Print and shaded views of the part. All mm, measured from the part's lowest x, y and z. A direction names the side the tool comes from. Round coordinates to 2 decimals unless told otherwise and drop trailing zeros. Write each loop counter-clockwise with the first axis right and the second up, starting at its lowest first coordinate (ties: lowest second). Pieces come first, ordered by that corner, then holes. Notation, with made-up numbers: (5, -5) - (22, -5) arc R15 ccw to (22, 18) - close; hole circle Ø10 at (56, 84). An arc over 180 degrees is marked (long way). Put each result on its own line as item: value. Start each with the question number.
Item 1: Drill centre lines: line 1 (X direction, y = 5.25, z = 1.25); line 2 (Z direction, x = 8, y = 4.25) (3 decimals); line 3 (Y direction, x = 5.25, z = 7.25). Where is each one in solid material? Low to high. Write a range as from..to.
Item 2: 3-axis set-ups, long thin cutter, end or side, ignore diameter. For the marked faces 1 and 2: which of +Z, -Z, +X, -X, +Y, -Y reach the whole face in a straight line?
Item 3: Cut at C-C (z = 2.75). Give the cut face in (x, y).
Item 4: Cut at D-D (z = 13). Give the cut face in (x, y) (3 decimals), and give its area (3 significant figures).
Item 5: Cut at A-A (x = 5.08). Give the cut face in (y, z) (3 decimals), and give its area (3 significant figures).
Item 6: Pin check, flat tips, straight feed: pin 1 Ø1.5 at (y, z) = (6, 7.5) entering from -X; pin 2 Ø6 at (x, y) = (3, 8.5) entering from +Z (3 decimals); pin 3 Ø1.5 at (y, z) = (7, 3) entering from +X; pin 4 Ø6 at (x, z) = (5.5, 11.5) entering from -Y (3 decimals). Stop position of each tip, or through.
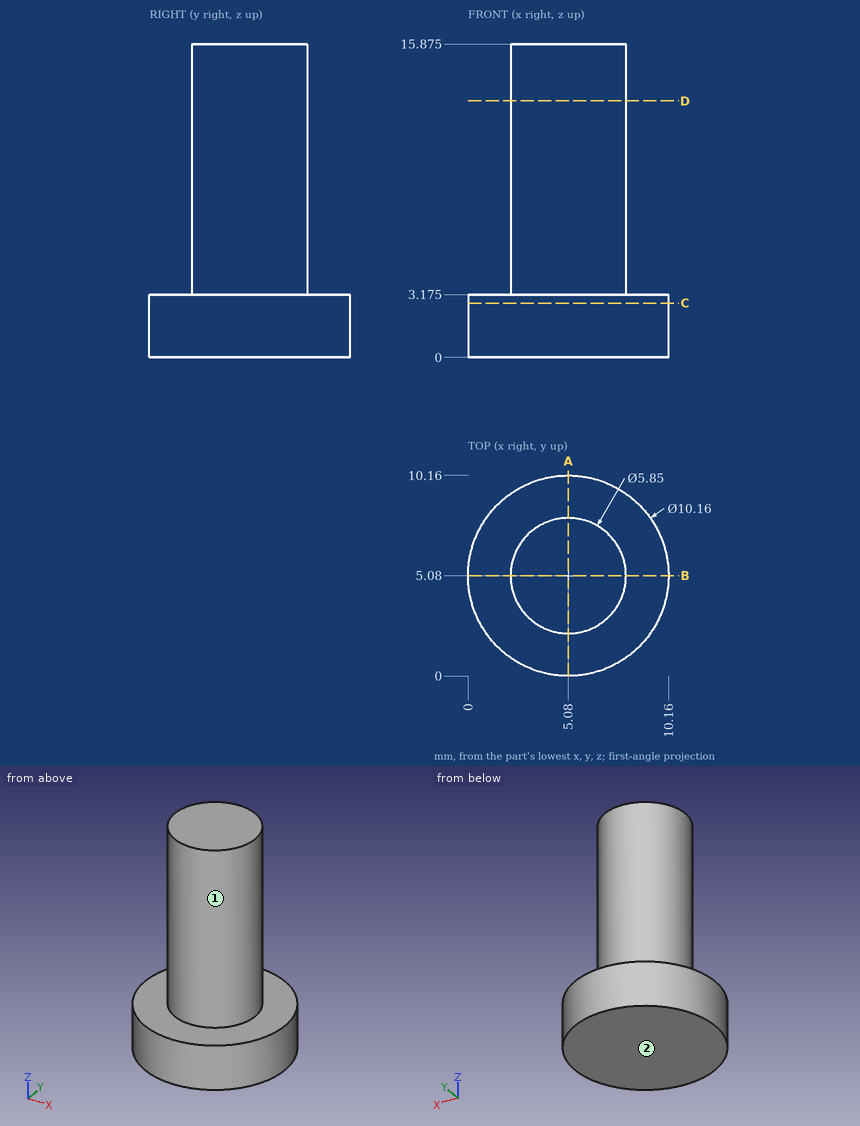
Output values:
1. line 1: 0..10.16
1. line 2: 0..3.175
1. line 3: 2.16..8
2. face 1: +Z
2. face 2: -Z, +X, -X, +Y, -Y
3. outline: circle Ø10.16 at (5.08, 5.08)
4. outline: circle Ø5.85 at (5.08, 5.08)
4. area: 26.9 mm2
5. outline: (0, 0) - (10.16, 0) - (10.16, 3.175) - (8.005, 3.175) - (8.005, 15.875) - (2.155, 15.875) - (2.155, 3.175) - (0, 3.175) - close
5. area: 107 mm2
6. pin 1: x = 2.16
6. pin 2: z = 15.875
6. pin 3: x = 10.02
6. pin 4: y = 2.155
